Design review of the part built by this model. Coordinates are the model's own, in mm. Give positions to 0.01 mm unless a question says otherwise; leave off trailing zeros. Order: outer loops, then holes, each group sorted by start corner. A loop starts at its lowest first (then second) coordinate and runs counter-clockwise, first axis right, second up. Notation, with made-up numbers: (11, 63.5) -> (19, 63.5) arc R19 cw to (19, 96.5) -> close; hole circle Ø3 at (-26, 68). An arc over 180 degrees is marked (long way). One line per item, written item: value. Start each with the question number.
1) For pin 1 (0.9 mm diameter, centred on y = 92, z = 4, fed in from -X); pin 2 (2.5 mm diameter, centred on y = 53, z = 4.5, fed in from +X), all flat-tipped, find the tip position at first contact; note any pin that passes through.
2) Consider section B-B (y = 167.5). State the section outline as (x, z) points, plus the area to 3 significant figures.
3) Wall thickness on line 1 along Z through (x, y) = (-18, 137); line 2 along X through (y, z) = (135.5, 5); line 3 along X through (y, z) = (80.5, -6.25): over which ranges is each line inside the solid? List them lowest first. Write a range as from..to.
4) Consider section A-A (x = -19.5). State the section outline as (y, z) points.
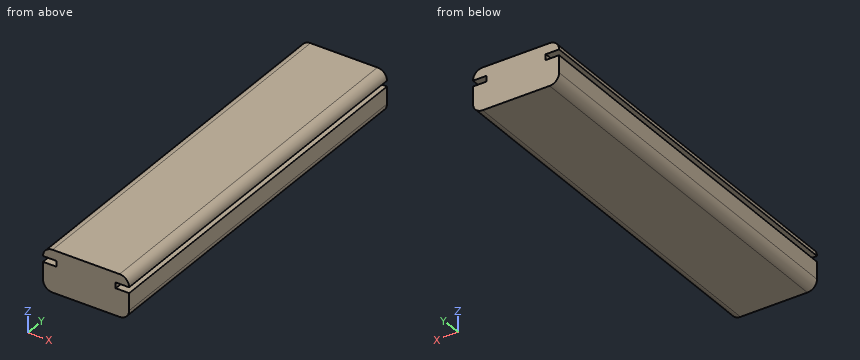
from build123d import *

# Parameters (mm, degrees)
F0_W     = 45
F0_H     = 22
F1_DEPTH = 200
F2_R     = 5
F3_W     = 200
F3_H     = 3
F4_DEPTH = 7
F5_W     = 200
F5_H     = 3
F6_DEPTH = 7


with BuildPart() as f1:
    # F0 (on Front) → F1 (new body)
    with BuildSketch(Plane.XZ):
        Rectangle(F0_W, F0_H)
    extrude(amount=-F1_DEPTH)

    # F2
    f2_edges = [f1.edges().sort_by_distance(p)[0] for p in [
        (22.5, 100, 11),
        (-22.5, 100, 11),
        (22.5, 100, -11),
        (-22.5, 100, -11),
    ]]
    fillet(f2_edges, radius=F2_R)

    # F3 (on face) → F4 (cut)
    with BuildSketch(Plane.YZ.offset(22.5)):
        with Locations((100, 4.5)):
            Rectangle(F3_W, F3_H)
    extrude(amount=-F4_DEPTH, mode=Mode.SUBTRACT)

    # F5 (on face) → F6 (cut)
    with BuildSketch(Plane(origin=(-22.5, 0, 0), x_dir=(0, -1, 0), z_dir=(-1, 0, 0))):
        with Locations((-100, 4.5)):
            Rectangle(F5_W, F5_H)
    extrude(amount=-F6_DEPTH, mode=Mode.SUBTRACT)


solid = f1.part
Checked values:
1. pin 1: stops at x = -15.5
1. pin 2: stops at x = 15.5
2. outline: (-22.5, -6) arc R5 ccw to (-17.5, -11) -> (17.5, -11) arc R5 ccw to (22.5, -6) -> (22.5, 3) -> (15.5, 3) -> (15.5, 6) -> (22.5, 6) arc R5 ccw to (17.5, 11) -> (-17.5, 11) arc R5 ccw to (-22.5, 6) -> (-15.5, 6) -> (-15.5, 3) -> (-22.5, 3) -> close
2. area: 927 mm^2
3. line 1: z = -10.97..3, 6..10.97
3. line 2: x = -15.5..15.5
3. line 3: x = -22.49..22.49
4. outline: (0, -10.58) -> (200, -10.58) -> (200, 3) -> (0, 3) -> close; (0, 6) -> (200, 6) -> (200, 10.58) -> (0, 10.58) -> close
